Can you work these out from the drawing? Everything is in mm from the part's minimum corner. A direction names the side the tool comes from. Give positions to 0.01 mm unless a question says otherwise; leave off trailing zeros. Write each loop counter-clockwise with the first axis right and the second up, starting at its lowest first coordinate (ties: lowest second). Pieces come first, ordered by that corner, then holes. Notation, with made-up numbers: (-22.75, 51.5) -> (-17.75, 51.5) arc R26 cw to (-17.75, 76.5) -> close; hole circle Ø2 at (21, 75.5). An arc over 180 degrees is marked (long way). Use one line per item in the form item = value.
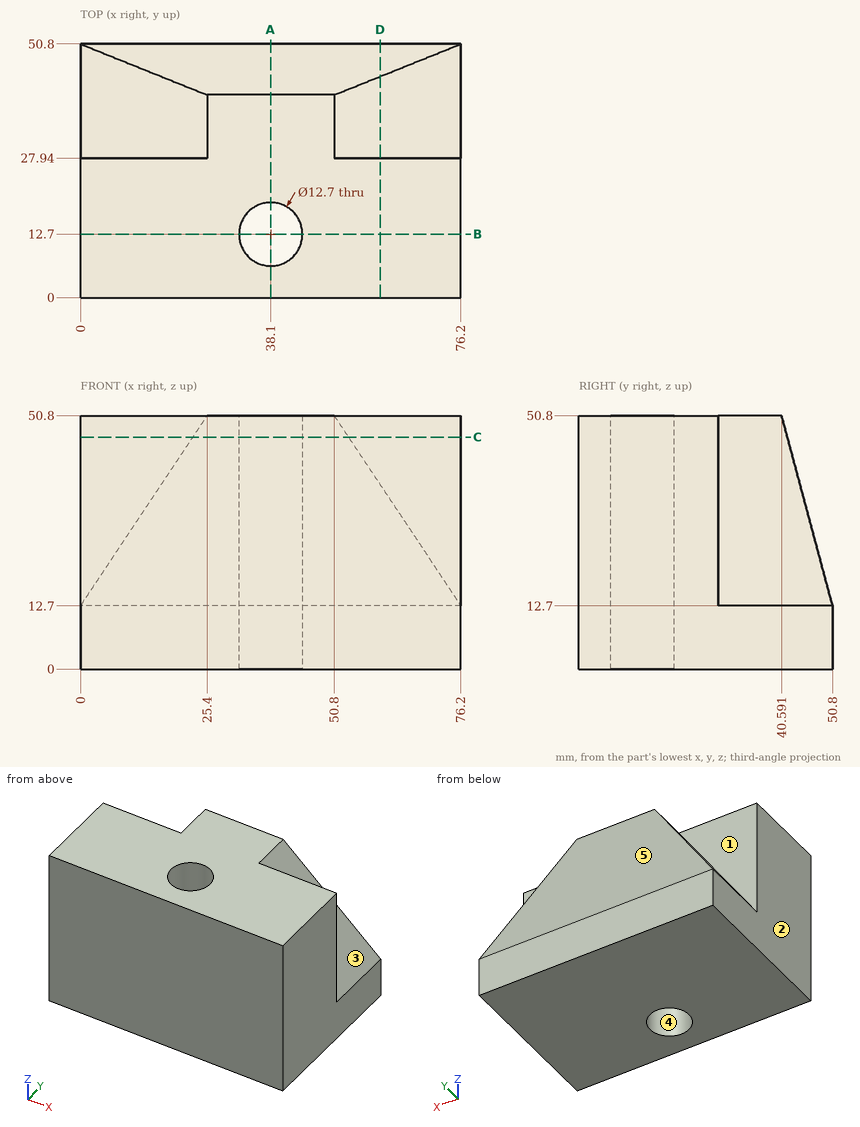
Q1. I want a section at D-D, the plane x = 60. Write out the boundary of the cut face in (y, z), and give its area (3 significant figures).
Result set:
outline = (0, 0) -> (50.8, 0) -> (50.8, 12.7) -> (44.29, 37) -> (27.94, 37) -> (27.94, 50.8) -> (0, 50.8) -> close
area = 2,190 mm2
Q2. I want a section at A-A, the plane x = 38.1. Write out the boundary of the cut face in (y, z), and give its area (3 significant figures).
Result set:
outline = (0, 0) -> (6.35, 0) -> (6.35, 50.8) -> (0, 50.8) -> close; (19.05, 0) -> (50.8, 0) -> (50.8, 12.7) -> (40.59, 50.8) -> (19.05, 50.8) -> close
area = 1,740 mm2
Q3. Will these pins go through, and if not, where does the flat tip stop? pin 1 Ø20.5 at (x, z) = (65, 28.5) entering from +Y; pin 2 Ø6 at (x, y) = (53, 42.5) entering from -Z; pin 3 Ø1.5 at (x, y) = (58.5, 41) entering from +Z (1 decimal).
Result set:
pin_1 = 49.31
pin_2 = 0
pin_3 = 40.4
Q4. Which directions (+Z, -Z, +X, -X, +Y, -Y) give clear straight access to the entire face, cutting with the end or side of a thin tool? Please do the marked faces 1 and 2.
Result set:
face_1 = +Z, -X, +Y
face_2 = +Z, -Z, -X, +Y, -Y
Q5. If we mould it in two halves opening along X, with no side actions, what happens to the marked faces 3, 4 and 5? For each: +X half, -X half, draft (parallel to the pull), parting line (faces both ways), or undercut.
Result set:
face_3 = +X half
face_4 = undercut
face_5 = draft
Q6. If I drill on line 1 along X through (y, z) = (12.5, 19); line 2 along Y through (x, z) = (38.5, 5); line 3 along Y through (x, z) = (39.5, 26.5), over which ranges is the centre line in solid material (lowest first)? Write a range as from..to.
Result set:
line_1 = 0..31.75, 44.45..76.2
line_2 = 0..6.36, 19.04..50.8
line_3 = 0..6.51, 18.89..47.1
Q7. I want a section at C-C, the plane z = 46.5. Write out the boundary of the cut face in (x, y).
Result set:
outline = (0, 0) -> (76.2, 0) -> (76.2, 27.94) -> (53.67, 27.94) -> (53.67, 41.74) -> (22.53, 41.74) -> (22.53, 27.94) -> (0, 27.94) -> close; hole circle Ø12.7 at (38.1, 12.7)
Q8. I want a section at B-B, the plane y = 12.7. Write out the boundary of the cut face in (x, z), and give its area (3 significant figures).
Result set:
outline = (0, 0) -> (31.75, 0) -> (31.75, 50.8) -> (0, 50.8) -> close; (44.45, 0) -> (76.2, 0) -> (76.2, 50.8) -> (44.45, 50.8) -> close
area = 3,230 mm2
